Solid Edge part; units mm, degrees
sketch "Sketch1" plane through (0, 0, 0) normal (0, 0, 1) x (1, 0, 0)
  line L0 (-1, -25) -> (1, -25)
  line L1 (1, -25) -> (1, 25)
  line L2 (1, 25) -> (-1, 25)
  line L3 (-1, 25) -> (-1, -25)
  line L4 (-25, -1) -> (25, -1)
  line L5 (25, -1) -> (25, 1)
  line L6 (25, 1) -> (-25, 1)
  line L7 (-25, 1) -> (-25, -1)
extrude "Protrusion1" add sketch "Sketch1" along normal mid plane 26
Verification items for the finished model (mm, model axes). A direction names the side the tool comes from. Round coordinates to 2 decimals unless told otherwise and drop trailing zeros. Write each loop counter-clockwise with the first axis right and the second up, starting at its lowest first coordinate (ties: lowest second). Pieces come first, ordered by that corner, then holes.
1. Section check A-A on z = 2.25. Enter the section's corners in (x, y), plus the area to 3 significant figures.
2. Gauge pin test, flat ends, axial feed: P1, Ø12, axis at y = -12.5, z = 0.5, coming from the -X side; P2, Ø3, axis at x = 3, z = -3.5, coming from the -Y side; P3, Ø7, axis at y = 19, z = 6.5, coming from the +X side. Record the tip position at first contact, or that the pin passes through.
3. Section check B-B on y = -9.5. Enter the section's corners in (x, z).
4. Scan line: L1, parallel to X at y = -9, z = -6.5. Record every from-to range of solid material in increasing order.
5. Access from +Z, -Z, +X, -X, +Y, -Y to the whole of each face (thin tool, end or side, straight path). Record for faces 1 (the flat face through (13, 1, 0)), 2 (the flat face through (-1, -13, 0)), 3 (the flat face through (-1, 13, 0)), 4 (the flat face through (13, -1, 0)).
Answer:
1. outline: (-25, -1) - (-1, -1) - (-1, -25) - (1, -25) - (1, -1) - (25, -1) - (25, 1) - (1, 1) - (1, 25) - (-1, 25) - (-1, 1) - (-25, 1) - close
1. area: 196 mm2
2. P1: stops at x = -1
2. P2: stops at y = -1
2. P3: stops at x = 1
3. outline: (-1, -13) - (1, -13) - (1, 13) - (-1, 13) - close
4. L1: x = -1 to 1
5. face 1: +Z, -Z, +X, +Y
5. face 2: +Z, -Z, -X, -Y
5. face 3: +Z, -Z, -X, +Y
5. face 4: +Z, -Z, +X, -Y
